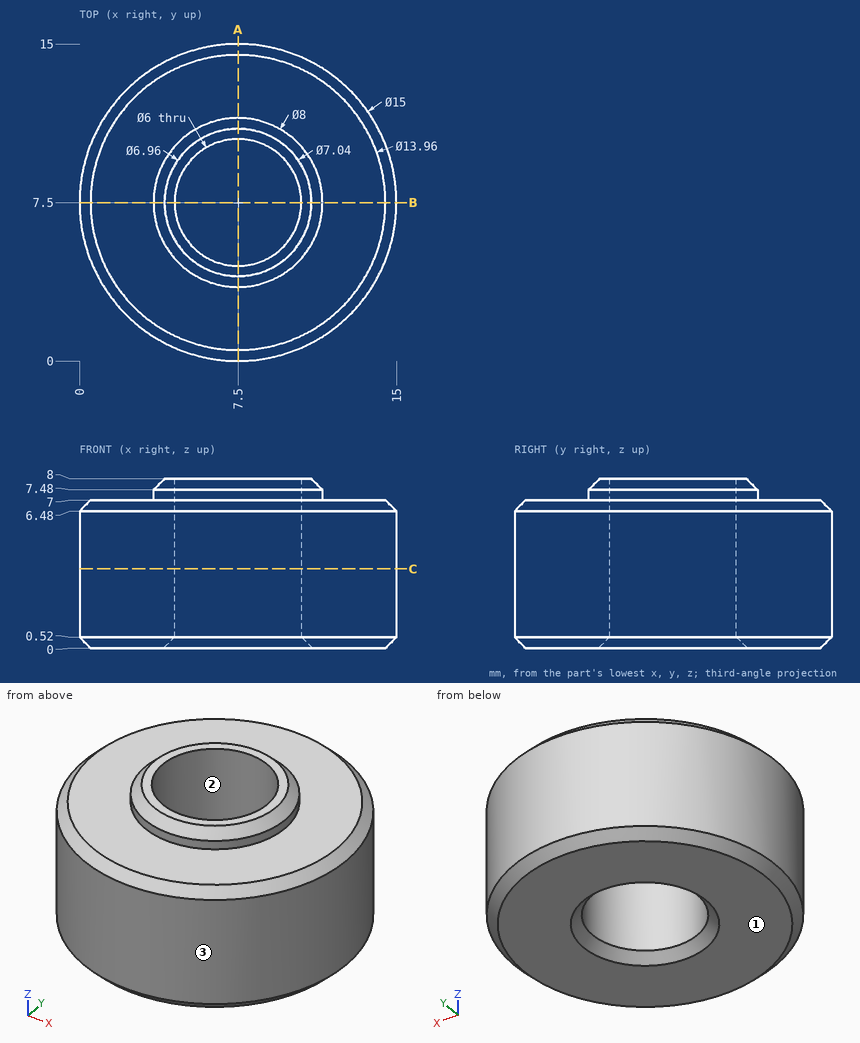
Job drawing, mm, ordinate dimensions from the low corner. One solid piece. Give positions to 0.01 mm unless a question says otherwise; leave off trailing zeros. Loops run counter-clockwise (first coordinate to the right, second up) from the corner with the lowest first, then second, coordinate; pieces in that order, holes last.
Item 1: Slice it at C-C, the plane z = 3.75. List the corners of the cut face in (x, y).
Answers follow:
outline: circle Ø15 at (7.5, 7.5); hole circle Ø6 at (7.5, 7.5)
Item 2: Flat gauge pin, fed straight in: pin 1 (1 mm diameter, centred on x = 13, z = 6, fed in from +Y). Where does the tip first touch, or does it go through?
Answers follow:
pin 1: stops at y = 13.09
Item 3: Pull direction Y, two halves, no side cores. Call the marked faces 1, 2 and 3: released by +Y, released by -Y, zero draft, split by the parting line, or undercut.
Answers follow:
face 1: zero draft
face 2: undercut
face 3: split by the parting line
Item 4: Slice it at A-A, the plane x = 7.5. List the corners of the cut face in (y, z).
Answers follow:
outline: (0, 0.52) - (0.52, 0) - (3.98, 0) - (4.5, 0.52) - (4.5, 8) - (4.02, 8) - (3.5, 7.48) - (3.5, 7) - (0.52, 7) - (0, 6.48) - close; (10.5, 0.52) - (11.02, 0) - (14.48, 0) - (15, 0.52) - (15, 6.48) - (14.48, 7) - (11.5, 7) - (11.5, 7.48) - (10.98, 8) - (10.5, 8) - close
Item 5: Drill centre lines: line 1 (Y direction, x = 7.5, z = 3); line 2 (Z direction, x = 14.25, y = 6.25); line 3 (X direction, y = 8.75, z = 6.25). Where is each one in solid material? Low to high.
Answers follow:
line 1: y = 0 to 4.5, 10.5 to 15
line 2: z = 0 to 7
line 3: x = 0.1 to 4.77, 10.23 to 14.9
